from build123d import *

# Parameters (mm, degrees)
BOSS_EXTRUDE6_DEPTH      = 100
BOSS_EXTRUDE6_DEPTH_BACK = 0.001
SKETCH19_R               = 6.25
SIDE_BUTTON_DEPTH        = 10
SKETCH21_W               = 13
SKETCH21_H               = 3
SD_DEPTH                 = 10
SKETCH_5_W               = 55
SKETCH_5_H               = 100.001
CUT_EXTRUDE_4_DEPTH      = 7
SKETCH_4_R               = 4
PORTS_DEPTH              = 1
TOP_COVER_DEPTH          = 1
SKETCH_7_W               = 30
SKETCH_7_H               = 2
EXTRUDE_5_DEPTH          = 30


with BuildPart() as part:
    # Sketch11 → Boss-Extrude6 (new, two sides: drawn at the far end of the back side and taken through both)
    with BuildSketch(Plane.XY.offset(-BOSS_EXTRUDE6_DEPTH_BACK)):
        with BuildLine():
            Line((-50.925767273, 31.436762529), (4.074232727, 31.436762529))
            ThreePointArc((4.074232727, 31.436762529), (16.843059589, 14.983457432), (13.439015431, -5.563237471))
            Line((13.439015431, -5.563237471), (-51.560984569, -5.563237471))
            ThreePointArc((-51.560984569, -5.563237471), (-58.976171577, 13.069519435), (-50.925767273, 31.436762529))
        make_face()
        with BuildLine():
            Line((-51.012961367, 30.835508878), (3.987038633, 30.835508878))
            ThreePointArc((3.987038633, 30.835508878), (15.684365135, 14.996890968), (13.439015431, -4.564491122))
            Line((13.439015431, -4.564491122), (-51.560984569, -4.564491122))
            ThreePointArc((-51.560984569, -4.564491122), (-57.931377732, 13.23837012), (-51.012961367, 30.835508878))
        make_face(mode=Mode.SUBTRACT)
    extrude(amount=BOSS_EXTRUDE6_DEPTH + BOSS_EXTRUDE6_DEPTH_BACK)

    # Sketch19 → side button (cut)
    with BuildSketch(Plane(origin=(17.637860169, 0, 0), x_dir=(0, 0, -1), z_dir=(1, 0, 0))):
        with Locations(Location((-55.2, 17.436762529, 0), (0, 0, 90))):
            Circle(SKETCH19_R)
    extrude(amount=-SIDE_BUTTON_DEPTH, mode=Mode.SUBTRACT)

    # Sketch21 → sd (cut)
    with BuildSketch(Plane.ZY.offset(58.980002369)):
        with Locations((62, -1.563237471)):
            Rectangle(SKETCH21_W, SKETCH21_H)
    extrude(amount=-SD_DEPTH, mode=Mode.SUBTRACT)

    # 草图5 → 切除-拉伸4 (cut)
    with BuildSketch(Plane(origin=(0, 31.436762529, 0), x_dir=(1, 0, 0), z_dir=(0, 1, 0))):
        with Locations((-23.425767273, -49.9995)):
            Rectangle(SKETCH_5_W, SKETCH_5_H)
    extrude(amount=-CUT_EXTRUDE_4_DEPTH, mode=Mode.SUBTRACT)

    # 草图4 → ports (add)
    with BuildSketch(Plane.XY.offset(100)):
        with BuildLine():
            Line((-50.925767273, 31.436762529), (4.074232727, 31.436762529))
            ThreePointArc((4.074232727, 31.436762529), (16.797971673, 14.972045579), (13.439015431, -5.563237471))
            Line((13.439015431, -5.563237471), (-51.560984569, -5.563237471))
            ThreePointArc((-51.560984569, -5.563237471), (-58.825710556, 13.066936315), (-50.925767273, 31.436762529))
        make_face()
        with Locations((-38.060984569, 11.436762529)):
            Circle(SKETCH_4_R, mode=Mode.SUBTRACT)
        with BuildLine():
            Line((-37.560984569, 1.332835104), (-27.101744103, 1.332835104))
            Line((-27.101744103, 1.332835104), (-27.101744103, -1.446793765))
            ThreePointArc((-27.101744103, -1.446793765), (-27.522930097, -1.907180738), (-28.029632197, -2.271332887))
            Line((-28.029632197, -2.271332887), (-37.028696773, -2.271332887))
            ThreePointArc((-37.028696773, -2.271332887), (-37.327749623, -1.880307962), (-37.560984569, -1.446793765))
            Line((-37.560984569, -1.446793765), (-37.560984569, 1.332835104))
        make_face(mode=Mode.SUBTRACT)
    extrude(amount=PORTS_DEPTH)

    # 草图6 → top cover (add)
    with BuildSketch(Plane(origin=(0, 0, -0.001), x_dir=(-1, 0, 0), z_dir=(0, 0, -1))):
        with BuildLine():
            Line((-4.074232727, 31.436762529), (50.925767273, 31.436762529))
            ThreePointArc((50.925767273, 31.436762529), (58.934474425, 13.068803577), (51.560984569, -5.563237471))
            Line((51.560984569, -5.563237471), (-13.439015431, -5.563237471))
            ThreePointArc((-13.439015431, -5.563237471), (-16.680513275, 14.942316596), (-4.074232727, 31.436762529))
        make_face()
    extrude(amount=TOP_COVER_DEPTH)

    # 草图7 → 凸台-拉伸5 (add)
    with BuildSketch(Plane(origin=(0, -4.564491122, 0), x_dir=(1, 0, 0), z_dir=(0, 1, 0))):
        with Locations((-19.060984569, -29)):
            Rectangle(SKETCH_7_W, SKETCH_7_H)
    extrude(amount=EXTRUDE_5_DEPTH)


solid = part.part
Can you work these out from the model? Positions are in its coordinate system, mm. A direction names the side the tool comes from. Coordinates: 2 decimals unless noted, no trailing zeros. Loops run counter-clockwise (first coordinate to the right, second up) from the corner with the lowest first, then second, coordinate; pieces in that order, holes last. Notation, with made-up numbers: (-14, 21.5) - (-10, 21.5) arc R27 ccw to (-10, 45.5) - close; hole circle Ø2 at (-7.75, -7). An arc over 180 degrees is marked (long way). Put each result on its own line as item: value. Start each with the question number.
Item 1: Suppose I cut it at A-A (z = 35). Please give me the cut outline in (x, y).
Item 2: Suppose I cut it at B-B (x = -44). Please give me the cut outline in (y, z), and give its area (3 significant figures).
Item 3: If we mould it in two halves opening along Z, with no side actions, what happens to faces 1 (the face through (-21, 13, -1.001)), 2 (the face through (16.752, 14.652, -0.494)), 3 (the face through (-19, -4.564, 49))? For each: +Z half, -Z half, draft (parallel to the pull), parting line (faces both ways), or undercut.
Item 4: For pin 1 (0.6 mm diameter, centred on x = -16, z = 29, fed in from +Y); pin 2 (1.1 mm diameter, centred on y = 0.5, z = 100.5, fed in from -X); pin 3 (2 mm diameter, centred on y = 18, z = 22, fed in from -X), each with a flat end and sliding along its axis, tell me the tip position at first contact or that it passes through.
Item 5: Which directions (+Z, -Z, +X, -X, +Y, -Y) give clear straight access to the entire face, cutting with the end or side of a thin tool? Please do faces 4 (the face through (-42.057, 11.613, 100.493)), 5 (the face through (-54.2, -1.5, 68.5)), 6 (the face through (-19, 10, 30)), 7 (the face through (14.56, 20.48, 49.74)).
Item 6: If I drill on line 1 along Z through (x, y) = (-7.5, -3); line 2 along Z through (x, y) = (11, 6); line 3 along Y through (x, z) = (-16, 90.5), over which ranges is the centre line in solid material (lowest first)?
Item 7: Suppose I cut it at D-D (x = -6.5). Please give me the cut outline in (y, z), and give its area (3 significant figures).
Here are the results:
1. outline: (-51.56, -5.56) - (13.44, -5.56) arc R26 ccw to (4.07, 31.44) - (4.07, 30.78) arc R26.86 cw to (13.44, -4.56) - (-51.56, -4.56) arc R26.9 cw to (-51.01, 30.84) - (-50.93, 30.84) - (-50.93, 31.44) arc R26 ccw to start
2. outline: (-5.56, -1) - (31.44, -1) - (31.44, 0) - (-4.56, 0) - (-4.56, 100) - (31.44, 100) - (31.44, 101) - (-5.56, 101) - close
2. area: 174 mm²
3. face 1: -Z half
3. face 2: draft
3. face 3: undercut
4. pin 1: y = 25.44
4. pin 2: x = -56.16
4. pin 3: x = -58.61
5. face 4: +Z
5. face 5: -X
5. face 6: +Y
5. face 7: +X
6. line 1: -1 to 0, 28 to 30, 100 to 101
6. line 2: -1 to 0, 100 to 101
6. line 3: -5.56 to -4.56
7. outline: (-5.56, -1) - (31.44, -1) - (31.44, 0) - (-4.56, 0) - (-4.56, 28) - (25.44, 28) - (25.44, 30) - (-4.56, 30) - (-4.56, 100) - (31.44, 100) - (31.44, 101) - (-5.56, 101) - close
7. area: 234 mm²
